from build123d import *

# Parameters (mm, degrees)
SKETCH1_W           = 350.8375
SKETCH1_H           = 152.4
BOSS_EXTRUDE1_DEPTH = 2.38125
CUT_EXTRUDE1_DEPTH  = 5.7625


with BuildPart() as part:
    # Sketch1 → Boss-Extrude1 (new body, symmetric)
    with BuildSketch(Plane(origin=(0, 0, 0), x_dir=(1, 0, 0), z_dir=(0, 1, 0))):
        Rectangle(SKETCH1_W, SKETCH1_H)
    extrude(amount=BOSS_EXTRUDE1_DEPTH, both=True)

    # Sketch2 → Cut-Extrude1 (cut, through all)
    with BuildSketch(Plane(origin=(0, 2.38125, 0), x_dir=(1, 0, 0), z_dir=(0, 1, 0))):
        with BuildLine():
            Line((102.39375, 9.525), (83.34375, 9.525))
            ThreePointArc((83.34375, 9.525), (57.94375, 34.925), (83.34375, 60.325))
            Line((83.34375, 60.325), (102.39375, 60.325))
            ThreePointArc((102.39375, 60.325), (127.79375, 34.925), (102.39375, 9.525))
        make_face()
        with BuildLine():
            Line((-137.31875, 50.8), (-61.11875, 50.8))
            ThreePointArc((-61.11875, 50.8), (-49.385479937, 42.960079591), (-52.138493879, 29.119743879))
            Line((-52.138493879, 29.119743879), (-128.338493879, -47.080256121))
            ThreePointArc((-128.338493879, -47.080256121), (-142.178829591, -49.833270063), (-150.01875, -38.1))
            Line((-150.01875, -38.1), (-150.01875, 38.1))
            ThreePointArc((-150.01875, 38.1), (-146.299006121, 47.080256121), (-137.31875, 50.8))
        make_face()
        with BuildLine():
            Line((-65.476701031, -50.8), (10.723298969, -50.8))
            ThreePointArc((10.723298969, -50.8), (19.70355509, -47.080256121), (23.423298969, -38.1))
            Line((23.423298969, -38.1), (23.423298969, 38.1))
            ThreePointArc((23.423298969, 38.1), (15.58337856, 49.833270063), (1.743042847, 47.080256121))
            Line((1.743042847, 47.080256121), (-74.456957153, -29.119743879))
            ThreePointArc((-74.456957153, -29.119743879), (-77.209971094, -42.960079591), (-65.476701031, -50.8))
        make_face()
        with BuildLine():
            Line((61.523298969, -50.8), (137.31875, -50.8))
            ThreePointArc((137.31875, -50.8), (146.299006121, -47.080256121), (150.01875, -38.1))
            Line((150.01875, -38.1), (150.01875, -28.575))
            ThreePointArc((150.01875, -28.575), (146.299006121, -19.594743879), (137.31875, -15.875))
            Line((137.31875, -15.875), (61.523298969, -15.875))
            ThreePointArc((61.523298969, -15.875), (52.543042847, -19.594743879), (48.823298969, -28.575))
            Line((48.823298969, -28.575), (48.823298969, -38.1))
            ThreePointArc((48.823298969, -38.1), (52.543042847, -47.080256121), (61.523298969, -50.8))
        make_face()
    extrude(amount=-CUT_EXTRUDE1_DEPTH, mode=Mode.SUBTRACT)


solid = part.part
Geometry: final body of the model. Coordinates: model frame, mm. A direction names the side the tool comes from. Give positions to 0.01 mm unless a question says otherwise; leave off trailing zeros. Write each loop counter-clockwise with the first axis right and the second up, starting at its lowest first coordinate (ties: lowest second). Pieces come first, ordered by that corner, then holes.
(1) Cut plane A-A, the plane y = -0.3. Return loops of the section in (x, z) (1 decimal).
(2) Cut plane C-C, the plane z = 20. Return loops of the section in (x, y).
(3) Access query for faces 1 (the cylindrical face through (52.64, 0.03, 19.5)), 2 (the flat face through (37, -2.381, -1)). Directions: +Z, -Z, +X, -X, +Y, -Y. A direction counts if a zero-diameter tool reaches every point of the face in a straight line with its end or side. Return the directions, or none.
(4) Mould query, pull axis X, two halves, no side actions, for faces 3 (the cylindrical face through (127.788, 0.033, -35.484)), 4 (the flat face through (-35.824, 0.033, -9.514)), 5 (the flat face through (37, 2.381, -1)). Classes: released by +X, released by -X, zero draft, split by the parting line, or undercut.
(5) Ray query, line 1 (Z direction, x = 100.5, y = 2.05) (3 decimals); line 2 (Z direction, x = 79.5, y = 1.7) (3 decimals); line 3 (X direction, y = -0.25, z = -2). Return the intervals inside material, ascending.
(6) Cut plane B-B, the plane x = -91.5. Return loops of the section in (y, z).
(7) Cut plane D-D, the plane z = -1. Return loops of the section in (x, y), then the cut area to 3 significant figures.
Values follow:
1. outline: (-175.4, -76.2) - (175.4, -76.2) - (175.4, 76.2) - (-175.4, 76.2) - close; hole (-150, -38.1) arc R12.7 ccw to (-137.3, -50.8) - (-61.1, -50.8) arc R12.7 ccw to (-52.1, -29.1) - (-128.3, 47.1) arc R12.7 ccw to (-150, 38.1) - close; hole (-74.5, 29.1) - (1.7, -47.1) arc R12.7 ccw to (23.4, -38.1) - (23.4, 38.1) arc R12.7 ccw to (10.7, 50.8) - (-65.5, 50.8) arc R12.7 ccw to start; hole (48.8, 28.6) arc R12.7 ccw to (61.5, 15.9) - (137.3, 15.9) arc R12.7 ccw to (150, 28.6) - (150, 38.1) arc R12.7 ccw to (137.3, 50.8) - (61.5, 50.8) arc R12.7 ccw to (48.8, 38.1) - close; hole (83.3, -60.3) - (102.4, -60.3) arc R25.4 ccw to (102.4, -9.5) - (83.3, -9.5) arc R25.4 ccw to start
2. outline: (-175.42, -2.38) - (-150.02, -2.38) - (-150.02, 2.38) - (-175.42, 2.38) - close; (-101.26, -2.38) - (-65.34, -2.38) - (-65.34, 2.38) - (-101.26, 2.38) - close; (23.42, -2.38) - (52.16, -2.38) - (52.16, 2.38) - (23.42, 2.38) - close; (146.69, -2.38) - (175.42, -2.38) - (175.42, 2.38) - (146.69, 2.38) - close
3. face 1: +Y, -Y
3. face 2: +Z, -Z, +X, -X, -Y
4. face 3: undercut
4. face 4: undercut
4. face 5: zero draft
5. line 1: z = -76.2 to -60.325, -9.525 to 15.875, 50.8 to 76.2
5. line 2: z = -76.2 to -60.032, -9.818 to 15.875, 50.8 to 76.2
5. line 3: x = -175.42 to -150.02, -79.26 to -43.34, 23.42 to 175.42
6. outline: (-2.38, -76.2) - (2.38, -76.2) - (2.38, -50.8) - (-2.38, -50.8) - close; (-2.38, 10.24) - (2.38, 10.24) - (2.38, 76.2) - (-2.38, 76.2) - close
7. outline: (-175.42, -2.38) - (-150.02, -2.38) - (-150.02, 2.38) - (-175.42, 2.38) - close; (-80.26, -2.38) - (-44.34, -2.38) - (-44.34, 2.38) - (-80.26, 2.38) - close; (23.42, -2.38) - (175.42, -2.38) - (175.42, 2.38) - (23.42, 2.38) - close
7. area: 1,020 mm2
